Build history of the part. All positions in model axes, mm. A direction names the side the tool comes from. Coordinates: 2 decimals unless noted, no trailing zeros. Order: outer loops, then holes, each group sorted by start corner. A loop starts at its lowest first (then second) coordinate and runs counter-clockwise, first axis right, second up. Notation, with made-up numbers: M 75.25,76.25 L 133.25,76.25 A19 ccw 133.25,91.25 Z; hole C 87.5,-34.5 d7. An arc over 180 degrees is marked long. Use a Markdown table: item, result. Add a question column.
from build123d import *

# Parameters (mm, degrees)
BOSS_EXTRUDE1_START       = -0.808533663
BOSS_EXTRUDE1_DEPTH       = 0.808533663
BOSS_EXTRUDE1_START_2     = 0.611119732
BOSS_EXTRUDE1_2_OUTLINE_W = 1
BOSS_EXTRUDE1_2_OUTLINE_H = 6.35
BOSS_EXTRUDE1_2_DEPTH     = 15.249880268
BOSS_EXTRUDE1_3_OUTLINE_W = 1
BOSS_EXTRUDE1_3_OUTLINE_H = 3.970866667
BOSS_EXTRUDE1_3_DEPTH     = 0.80872757
BOSS_EXTRUDE1_4_OUTLINE_W = 1
BOSS_EXTRUDE1_4_OUTLINE_H = 2.379133333
BOSS_EXTRUDE1_4_DEPTH     = 0.204646605
BOSS_EXTRUDE1_START_3     = 2.175
BOSS_EXTRUDE1_5_DEPTH     = 6
BOSS_EXTRUDE1_START_4     = 12.448968436
BOSS_EXTRUDE1_6_OUTLINE_W = 5
BOSS_EXTRUDE1_6_OUTLINE_H = 8.175
BOSS_EXTRUDE1_6_DEPTH     = 1.551031564
BOSS_EXTRUDE2_START       = 5.35
BOSS_EXTRUDE2_DEPTH       = 5.35
CUT_EXTRUDE1_DEPTH        = 6.35
BOSS_EXTRUDE3_DEPTH       = 14.191466337
BOSS_EXTRUDE4_REACH       = 36.333
CUT_EXTRUDE2_DEPTH        = 6.35
CUT_EXTRUDE3_DEPTH        = 6.35
CUT_EXTRUDE4_DEPTH        = 6.35
CUT_EXTRUDE5_DEPTH        = 6.35
CUT_EXTRUDE6_DEPTH        = 6.35
CUT_EXTRUDE7_DEPTH        = 41.809385627
CUT_EXTRUDE8_DEPTH        = 41.809385627
CUT_EXTRUDE9_DEPTH        = 41.809385627
SKETCH15_W                = 4.2
SKETCH15_H                = 12.2
CUT_EXTRUDE10_DEPTH       = 43.984969129
F_3_CLEARANCE_HOLE1_D     = 2
F_3_CLEARANCE_HOLE1_DEPTH = 30.861103078


with BuildPart() as part:
    # Boss-Extrude1: read off the stored shape, not the designer's step
    # Boss-Extrude1 outline → Boss-Extrude1 (new body)
    with BuildSketch(Plane(origin=(-0.4305, 0, 0), x_dir=(0, 0, -1), z_dir=(1, 0, 0)).offset(BOSS_EXTRUDE1_START)):
        Polygon((-11.175, -0.175), (-8.175, -3.175), (-2.175, -3.175), (-2.175, 28.325), (-8.175, 28.325), (-11.175, 25.325), align=None)
    extrude(amount=BOSS_EXTRUDE1_DEPTH)



with BuildPart() as body_2:
    # Boss-Extrude1 2 outline → Boss-Extrude1 2 (new body)
    with BuildSketch(Plane(origin=(-0.4305, 0, 0), x_dir=(0, 0, -1), z_dir=(1, 0, 0)).offset(BOSS_EXTRUDE1_START_2)):
        with Locations((-2.675, 0)):
            Rectangle(BOSS_EXTRUDE1_2_OUTLINE_W, BOSS_EXTRUDE1_2_OUTLINE_H)
    extrude(amount=BOSS_EXTRUDE1_2_DEPTH)


with BuildPart() as part_1:
    add(part.part)

    add(body_2.part)  # Boss-Extrude1 3 merges body 2
    # Boss-Extrude1 3 outline → Boss-Extrude1 3 (add)
    with BuildSketch(Plane(origin=(-0.4305, 0, 0), x_dir=(0, 0, -1), z_dir=(1, 0, 0))):
        with Locations((-2.675, -1.189566667)):
            Rectangle(BOSS_EXTRUDE1_3_OUTLINE_W, BOSS_EXTRUDE1_3_OUTLINE_H)
    extrude(amount=BOSS_EXTRUDE1_3_DEPTH)

    # Boss-Extrude1 4 outline → Boss-Extrude1 4 (add)
    with BuildSketch(Plane(origin=(-0.4305, 0, 0), x_dir=(0, 0, -1), z_dir=(1, 0, 0))):
        with Locations((-2.675, 1.985433334)):
            Rectangle(BOSS_EXTRUDE1_4_OUTLINE_W, BOSS_EXTRUDE1_4_OUTLINE_H)
    extrude(amount=BOSS_EXTRUDE1_4_DEPTH)

    # Boss-Extrude1 5 outline → Boss-Extrude1 5 (cut)
    with BuildSketch(Plane.XY.offset(BOSS_EXTRUDE1_START_3)):
        with BuildLine():
            Line((0.37822757, 0.934233164), (1.1938, 3.175))
            Line((1.1938, 3.175), (0.180619732, 3.175))
            Line((0.180619732, 3.175), (0.180619732, 0.795866667))
            ThreePointArc((0.180619732, 0.795866667), (0.301237045, 0.83389716), (0.37822757, 0.934233164))
        make_face()
        Polygon((15.385266337, 3.175), (15.4305, 3.050721534), (15.4305, 3.175), align=None)
        with BuildLine():
            Line((-0.4305, 0.953572019), (-0.423461232, 0.934233164))
            ThreePointArc((-0.423461232, 0.934233164), (-0.346470708, 0.83389716), (-0.225853395, 0.795866667))
            Line((-0.225853395, 0.795866667), (-0.225853395, 3.175))
            Line((-0.225853395, 3.175), (-0.4305, 3.175))
            Line((-0.4305, 3.175), (-0.4305, 0.953572019))
        make_face()
    extrude(amount=BOSS_EXTRUDE1_5_DEPTH, mode=Mode.SUBTRACT)

    # Boss-Extrude1 6 outline → Boss-Extrude1 6 (cut)
    with BuildSketch(Plane(origin=(0, 0, 0), x_dir=(0.707106781186545, 0, -0.70710678118655), z_dir=(0.70710678118655, 0, 0.707106781186545)).offset(BOSS_EXTRUDE1_START_4)):
        with Locations((8.5, 0.9125)):
            Rectangle(BOSS_EXTRUDE1_6_OUTLINE_W, BOSS_EXTRUDE1_6_OUTLINE_H)
    extrude(amount=BOSS_EXTRUDE1_6_DEPTH, mode=Mode.SUBTRACT)

    # Sketch2 → Boss-Extrude2 (add)
    with BuildSketch(Plane(origin=(0, 0, 2.175), x_dir=(-1, 0, 0), z_dir=(0, 0, -1)).offset(BOSS_EXTRUDE2_START)):
        with BuildLine():
            Line((1.239033663, -3.175), (-15.4305, -3.175))
            Line((-15.4305, -3.175), (-15.4305, 3.050721534))
            Line((-15.4305, 3.050721534), (-15.385266337, 3.175))
            Line((-15.385266337, 3.175), (-1.1938, 3.175))
            Line((-1.1938, 3.175), (-0.37822757, 0.934233164))
            ThreePointArc((-0.37822757, 0.934233164), (-0.301237046, 0.83389716), (-0.180619732, 0.795866667))
            Line((-0.180619732, 0.795866667), (0.225853395, 0.795866667))
            ThreePointArc((0.225853395, 0.795866667), (0.346470708, 0.83389716), (0.423461232, 0.934233164))
            Line((0.423461232, 0.934233164), (0.4305, 0.953572019))
            Line((0.4305, 0.953572019), (0.4305, 28.325))
            Line((0.4305, 28.325), (1.239033663, 28.325))
            Line((1.239033663, 28.325), (1.239033663, -3.175))
        make_face()
    extrude(amount=-BOSS_EXTRUDE2_DEPTH)

    # Sketch3 → Cut-Extrude1 (cut)
    with BuildSketch(Plane(origin=(0, 0, -3.175), x_dir=(-1, 0, 0), z_dir=(0, 0, -1))):
        Polygon((0.4305, 0.953572019), (1.239033663, 3.175), (1.239033663, 28.325), (0.4305, 28.325), align=None)
    extrude(amount=-CUT_EXTRUDE1_DEPTH, mode=Mode.SUBTRACT)

    # Sketch4 → Boss-Extrude3 (add)
    with BuildSketch(Plane.ZY.offset(1.239033663)):
        Polygon((3.175, 3.175), (3.175, 28.325), (8.175, 28.325), (11.175, 25.325), (11.175, -0.175), (8.175, -3.175), (-3.175, -3.175), (-3.175, 3.175), align=None)
    extrude(amount=BOSS_EXTRUDE3_DEPTH)

    # Boss-Extrude4: up to this plane
    boss_extrude4_end = Plane(origin=(-15.488026312, 0, 7.554015165), z_dir=(-0.8987940462991697, 0, 0.438371146789072))
    # Sketch6 → Boss-Extrude4 (add, up to the surface)
    with BuildSketch(Plane(origin=(-0.4305, 0, 0), x_dir=(0, 0, -1), z_dir=(1, 0, 0)), mode=Mode.PRIVATE) as boss_extrude4_sk1:
        with BuildLine():
            Line((-11.175, 1.575), (-11.175, 23.575))
            ThreePointArc((-11.175, 23.575), (-11.760786438, 22.160786438), (-13.175, 21.575))
            Line((-13.175, 21.575), (-28.175, 21.575))
            Line((-28.175, 21.575), (-28.175, 3.575))
            Line((-28.175, 3.575), (-13.175, 3.575))
            ThreePointArc((-13.175, 3.575), (-11.760786438, 2.989213562), (-11.175, 1.575))
        make_face()
    boss_extrude4_tool1 = split(extrude(boss_extrude4_sk1.sketch, amount=-BOSS_EXTRUDE4_REACH, mode=Mode.PRIVATE), bisect_by=boss_extrude4_end, keep=Keep.BOTH, mode=Mode.PRIVATE)
    add(boss_extrude4_tool1.solids().sort_by_distance((-0.4305, 12.575, 19.630069))[0])

    # Sketch7 → Cut-Extrude2 (cut)
    with BuildSketch(Plane(origin=(0, 0, -3.175), x_dir=(-1, 0, 0), z_dir=(0, 0, -1))):
        with BuildLine():
            Line((2.13106, 3.175), (2.94663243, 0.934233164))
            ThreePointArc((2.94663243, 0.934233164), (3.023622954, 0.83389716), (3.144240268, 0.795866667))
            Line((3.144240268, 0.795866667), (3.550713395, 0.795866667))
            ThreePointArc((3.550713395, 0.795866667), (3.671330708, 0.83389716), (3.748321232, 0.934233164))
            Line((3.748321232, 0.934233164), (4.563893663, 3.175))
            Line((4.563893663, 3.175), (2.13106, 3.175))
        make_face()
    extrude(amount=-CUT_EXTRUDE2_DEPTH, mode=Mode.SUBTRACT)

    # Sketch8 → Cut-Extrude3 (cut)
    with BuildSketch(Plane(origin=(0, 0, -3.175), x_dir=(-1, 0, 0), z_dir=(0, 0, -1))):
        with BuildLine():
            Line((5.45592, 3.175), (6.27149243, 0.934233164))
            ThreePointArc((6.27149243, 0.934233164), (6.348482954, 0.83389716), (6.469100268, 0.795866667))
            Line((6.469100268, 0.795866667), (6.875573395, 0.795866667))
            ThreePointArc((6.875573395, 0.795866667), (6.996190708, 0.83389716), (7.073181232, 0.934233164))
            Line((7.073181232, 0.934233164), (7.888753663, 3.175))
            Line((7.888753663, 3.175), (5.45592, 3.175))
        make_face()
    extrude(amount=-CUT_EXTRUDE3_DEPTH, mode=Mode.SUBTRACT)

    # Sketch9 → Cut-Extrude4 (cut)
    with BuildSketch(Plane(origin=(0, 0, -3.175), x_dir=(-1, 0, 0), z_dir=(0, 0, -1))):
        with BuildLine():
            Line((8.78078, 3.175), (9.59635243, 0.934233164))
            ThreePointArc((9.59635243, 0.934233164), (9.673342954, 0.83389716), (9.793960268, 0.795866667))
            Line((9.793960268, 0.795866667), (10.200433395, 0.795866667))
            ThreePointArc((10.200433395, 0.795866667), (10.321050708, 0.83389716), (10.398041232, 0.934233164))
            Line((10.398041232, 0.934233164), (11.213613663, 3.175))
            Line((11.213613663, 3.175), (8.78078, 3.175))
        make_face()
    extrude(amount=-CUT_EXTRUDE4_DEPTH, mode=Mode.SUBTRACT)

    # Sketch10 → Cut-Extrude5 (cut)
    with BuildSketch(Plane(origin=(0, 0, -3.175), x_dir=(-1, 0, 0), z_dir=(0, 0, -1))):
        with BuildLine():
            Line((12.10564, 3.175), (12.92121243, 0.934233164))
            ThreePointArc((12.92121243, 0.934233164), (12.998202954, 0.83389716), (13.118820268, 0.795866667))
            Line((13.118820268, 0.795866667), (13.525293395, 0.795866667))
            ThreePointArc((13.525293395, 0.795866667), (13.645910708, 0.83389716), (13.722901232, 0.934233164))
            Line((13.722901232, 0.934233164), (14.538473663, 3.175))
            Line((14.538473663, 3.175), (12.10564, 3.175))
        make_face()
    extrude(amount=-CUT_EXTRUDE5_DEPTH, mode=Mode.SUBTRACT)

    # Sketch11 → Cut-Extrude6 (cut)
    with BuildSketch(Plane(origin=(0, 0, -3.175), x_dir=(-1, 0, 0), z_dir=(0, 0, -1))):
        with BuildLine():
            Line((-12.060406337, 3.175), (-14.49324, 3.175))
            Line((-14.49324, 3.175), (-13.67766757, 0.934233164))
            ThreePointArc((-13.67766757, 0.934233164), (-13.600677046, 0.83389716), (-13.480059732, 0.795866667))
            Line((-13.480059732, 0.795866667), (-13.073586605, 0.795866667))
            ThreePointArc((-13.073586605, 0.795866667), (-12.952969292, 0.83389716), (-12.875978768, 0.934233164))
            Line((-12.875978768, 0.934233164), (-12.060406337, 3.175))
        make_face()
    extrude(amount=-CUT_EXTRUDE6_DEPTH, mode=Mode.SUBTRACT)

    # Sketch12 → Cut-Extrude7 (cut, through all)
    with BuildSketch(Plane.XY.offset(3.175)):
        with BuildLine():
            Line((2.085826337, 3.175), (2.901398768, 0.934233164))
            ThreePointArc((2.901398768, 0.934233164), (2.978389292, 0.83389716), (3.099006605, 0.795866667))
            Line((3.099006605, 0.795866667), (3.505479732, 0.795866667))
            ThreePointArc((3.505479732, 0.795866667), (3.626097046, 0.83389716), (3.70308757, 0.934233164))
            Line((3.70308757, 0.934233164), (4.51866, 3.175))
            Line((4.51866, 3.175), (2.085826337, 3.175))
        make_face()
    extrude(amount=-CUT_EXTRUDE7_DEPTH, mode=Mode.SUBTRACT)

    # Sketch13 → Cut-Extrude8 (cut, through all)
    with BuildSketch(Plane.XY.offset(3.175)):
        with BuildLine():
            Line((5.410686337, 3.175), (6.226258768, 0.934233164))
            ThreePointArc((6.226258768, 0.934233164), (6.303249292, 0.83389716), (6.423866605, 0.795866667))
            Line((6.423866605, 0.795866667), (6.830339732, 0.795866667))
            ThreePointArc((6.830339732, 0.795866667), (6.950957046, 0.83389716), (7.02794757, 0.934233164))
            Line((7.02794757, 0.934233164), (7.84352, 3.175))
            Line((7.84352, 3.175), (5.410686337, 3.175))
        make_face()
    extrude(amount=-CUT_EXTRUDE8_DEPTH, mode=Mode.SUBTRACT)

    # Sketch14 → Cut-Extrude9 (cut, through all)
    with BuildSketch(Plane.XY.offset(3.175)):
        with BuildLine():
            Line((8.735546337, 3.175), (9.551118768, 0.934233164))
            ThreePointArc((9.551118768, 0.934233164), (9.628109292, 0.83389716), (9.748726605, 0.795866667))
            Line((9.748726605, 0.795866667), (10.155199732, 0.795866667))
            ThreePointArc((10.155199732, 0.795866667), (10.275817046, 0.83389716), (10.35280757, 0.934233164))
            Line((10.35280757, 0.934233164), (11.16838, 3.175))
            Line((11.16838, 3.175), (8.735546337, 3.175))
        make_face()
    extrude(amount=-CUT_EXTRUDE9_DEPTH, mode=Mode.SUBTRACT)

    # Sketch15 → Cut-Extrude10 (cut, through all)
    with BuildSketch(Plane(origin=(-0.4305, 0, 0), x_dir=(0, 0, -1), z_dir=(1, 0, 0))):
        with Locations((-5.275, 12.575)):
            Rectangle(SKETCH15_W, SKETCH15_H)
    extrude(amount=-CUT_EXTRUDE10_DEPTH, mode=Mode.SUBTRACT)

    # #3 Clearance Hole1
    with Locations(Plane.ZY.offset(15.4305)):
        with Locations((6.675, 24.325), (6.675, 0.825)):
            Hole(F_3_CLEARANCE_HOLE1_D / 2, depth=F_3_CLEARANCE_HOLE1_DEPTH)


solid = part_1.part
(1) Drop flat-ended pins along their axis: P1, Ø1.5, axis at y = 15, z = 24, coming from the +X side; P2, Ø4, axis at y = 24.5, z = 19.5, coming from the +X side; P3, Ø1.9, axis at x = 5, y = 1, coming from the +Z side (3 decimals); P4, Ø3.5, axis at x = -7, y = 13.5, coming from the -Z side (3 decimals). Give the stop position or say it passes through.
(2) Slice it at D-D on z = 10.5. Give the cut face in (x, y), and give its area (3 significant figures).
(3) Mould opens along X. For faces 5 (the flat face through (-7.83, -1.65, 9.7)), 6 (the flat face through (-0.43, 12, 16)), 7 (the flat face through (9.138, 2.07, 0.044)) say: released by +X, released by -X, zero draft, split by the parting line, or undercut.
(4) Drill centre lines: line 1 along Y through (x, z) = (-6.5, 4.5) (3 decimals); line 2 along Z through (x, y) = (-4.5, 11.5) (3 decimals); line 3 along Y through (x, z) = (-3, 13). Where is each one in solid material? Low to high. Write a range as from..to.
(5) Slice it at B-B on y = 7. Give the cut face in (x, z) (1 decimal), and give its area (3 significant figures).
(6) Slice it at A-A on z = 6.5. Give the cut face in (x, y) (1 decimal), and give its area (3 significant figures).
(7) Which spindle directions (+Z, -Z, +X, -X, +Y, -Y) get a long thin tool onto all of the face, cutting with end or side? Do faces 1 (the flat face through (-8, 18.675, 5)), 2 (the flat face through (-4.15, 2.04, -0.04)), 3 (the flat face through (-8, 23, 3.175)), 4 (the flat face through (5.8, 2.1, 0)). Say none if no direction does.
(8) Slice it at C-C on z = 24.5. Give the cut face in (x, y) (1 decimal).
Solutions:
| question | item | result |
|---|---|---|
| 1 | P1 | x = -0.43 |
| 1 | P2 | through |
| 1 | P3 | z = 3.175 |
| 1 | P4 | z = 7.375 |
| 2 | outline | M -15.43,-0.85 L -0.43,-0.85 L -0.43,26 L -15.43,26 Z |
| 2 | area | 403 mm² |
| 3 | face 5 | zero draft |
| 3 | face 6 | released by +X |
| 3 | face 7 | undercut |
| 4 | line 1 | -3.175..6.475, 18.675..28.325 |
| 4 | line 2 | 7.375..28.175 |
| 4 | line 3 | 3.57..21.58 |
| 5 | outline | M -15.4,7.4 L -0.4,7.4 L -0.4,28.2 L -5.4,28.2 L -13.7,11.2 L -15.4,11.2 Z |
| 5 | area | 212 mm² |
| 6 | outline | M -15.4,-3.2 L -0.4,-3.2 L -0.4,-0.2 L -15.4,-0.2 Z; M -15.4,1.8 L -0.4,1.8 L -0.4,6.5 L -15.4,6.5 Z; M -15.4,18.7 L -0.4,18.7 L -0.4,23.3 L -15.4,23.3 Z; M -15.4,25.3 L -0.4,25.3 L -0.4,28.3 L -15.4,28.3 Z |
| 6 | area | 230 mm² |
| 7 | face 1 | -Z, +X, -X |
| 7 | face 2 | -Z, +Y |
| 7 | face 3 | -Z, +X, -X, +Y |
| 7 | face 4 | +Z, -Z, +Y |
| 8 | outline | M -7.2,3.6 L -0.4,3.6 L -0.4,21.6 L -7.2,21.6 Z |
